The listing builds one solid part. Answer for the finished solid, in the listing's coordinates (mm). Round coordinates to 2 decimals unless told otherwise and drop trailing zeros. Order: outer loops, then holes, each group sorted by start corner. A loop starts at its lowest first (then second) coordinate and runs counter-clockwise, first axis right, second up. Notation, with made-up numbers: M 77,-14.5 L 91,-14.5 A27 ccw 91,9.5 Z; hole C 37.5,-17 d2. An arc over 180 degrees is marked long. Put each result on its own line as item: value. Start each with the question number.
1. The part is cut by section B-B (x = 39.5). Give the vertices of the cut face in (y, z).
2. The part is cut by section C-C (z = 4). Give the vertices of the cut face in (x, y).
3. Consider line 1 (Z direction, x = -46, y = 14.85) (3 decimals); line 2 (Z direction, x = 62.5, y = 16.85); line 3 (X direction, y = 15.65, z = -12). Determine where each line is inside the solid, lowest interval first.
4. The part is cut by section A-A (x = -46). Give the vertices of the cut face in (y, z) (3 decimals), then the cut area to 4 significant figures.
5. Each of these flat-tipped pins is pushed along its axis until it touches: pin 1 Ø3 at (y, z) = (15, -4.5) entering from +X; pin 2 Ø1.8 at (x, z) = (62.5, -9) entering from +Y. Where does it stop, or does it pass through?
from build123d import *

# Parameters (mm, degrees)
BOSS_EXTRUDE1_DEPTH = 17.5
SKETCH2_W           = 18
SKETCH2_H           = 5
CUT_EXTRUDE1_DEPTH  = 17.5
SKETCH3_R           = 1.625
CUT_EXTRUDE2_DEPTH  = 5
SKETCH4_R           = 3
CUT_EXTRUDE3_DEPTH  = 2
CHAMFER1_SIZE       = 2


with BuildPart() as part:
    # Sketch1 → Boss-Extrude1 (new, symmetric)
    with BuildSketch(Plane.XY):
        with BuildLine():
            Line((-75, 17.5), (75, 17.5))
            ThreePointArc((75, 17.5), (81.614378278, 16.201851746), (87.247448714, 12.5))
            Line((87.247448714, 12.5), (-87.247448714, 12.5))
            ThreePointArc((-87.247448714, 12.5), (-81.614378278, 16.201851746), (-75, 17.5))
        make_face()
    extrude(amount=BOSS_EXTRUDE1_DEPTH, both=True)

    # Sketch2 → Cut-Extrude1 (cut, symmetric)
    with BuildSketch(Plane.XY):
        with Locations((-78.247448714, 15)):
            Rectangle(SKETCH2_W, SKETCH2_H)
    extrude(amount=CUT_EXTRUDE1_DEPTH, both=True, mode=Mode.SUBTRACT)

    # Sketch3 → Cut-Extrude2 (cut)
    with BuildSketch(Plane.XZ.offset(-12.5)):
        with Locations((-46, -10)):
            Circle(SKETCH3_R)
        with Locations((-9.833333333, -10)):
            Circle(SKETCH3_R)
        with Locations((26.333333333, -10)):
            Circle(SKETCH3_R)
        with Locations((62.5, -10)):
            Circle(SKETCH3_R)
    cut_extrude2 = extrude(amount=-CUT_EXTRUDE2_DEPTH, mode=Mode.SUBTRACT)

    # Sketch4 → Cut-Extrude3 (cut)
    with BuildSketch(Plane(origin=(0, 17.5, 0), x_dir=(1, 0, 0), z_dir=(0, 1, 0))):
        with Locations(Location((62.5, 9.8, 0), (0, 0, 180))):
            Circle(SKETCH4_R)
        with Locations(Location((26.333333333, 9.8, 0), (0, 0, 180))):
            Circle(SKETCH4_R)
        with Locations(Location((-9.833333333, 10, 0), (0, 0, 180))):
            Circle(SKETCH4_R)
        with Locations(Location((-46, 10, 0), (0, 0, 180))):
            Circle(SKETCH4_R)
    cut_extrude3 = extrude(amount=-CUT_EXTRUDE3_DEPTH, mode=Mode.SUBTRACT)

    # Mirror1: Cut-Extrude2, Cut-Extrude3 across plane
    add(cut_extrude2.mirror(Plane.XY), mode=Mode.SUBTRACT)
    add(cut_extrude3.mirror(Plane.XY), mode=Mode.SUBTRACT)

    # Chamfer1
    chamfer1_edges = [part.edges().sort_by_distance(p)[0] for p in [
        (81.614378278, 16.201851746, 17.5),
        (2.876275643, 17.5, 17.5),
        (2.876275643, 17.5, -17.5),
        (81.614378278, 16.201851746, -17.5),
    ]]
    chamfer(chamfer1_edges, length=CHAMFER1_SIZE)


solid = part.part
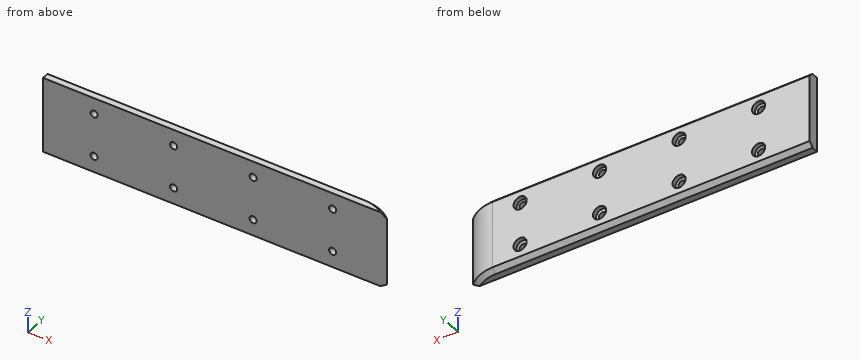
Resolved:
1. outline: M 12.5,-17.5 L 15.5,-17.5 L 17.5,-15.5 L 17.5,15.5 L 15.5,17.5 L 12.5,17.5 Z
2. outline: M -69.25,12.5 L 87.25,12.5 A17.5 ccw 75,17.5 L -69.25,17.5 Z
3. line 1: -17.5 to -11.625, -8.375 to 8.375, 11.625 to 17.5
3. line 2: -16.15 to -12.8, -6.8 to 6.8, 12.8 to 16.15
3. line 3: -69.25 to -48.24, -43.76 to -12.07, -7.6 to 24.29, 28.37 to 60.46, 64.54 to 82.83
4. outline: M 12.5,-17.5 L 15.5,-17.5 L 17.5,-15.5 L 17.5,-13 L 15.5,-13 L 15.5,-11.625 L 12.5,-11.625 Z; M 12.5,-8.375 L 15.5,-8.375 L 15.5,-7 L 17.5,-7 L 17.5,7 L 15.5,7 L 15.5,8.375 L 12.5,8.375 Z; M 12.5,11.625 L 15.5,11.625 L 15.5,13 L 17.5,13 L 17.5,15.5 L 15.5,17.5 L 12.5,17.5 Z
4. area: 127.5 mm2
5. pin 1: x = 86.14
5. pin 2: y = 15.5
